from build123d import *

# Parameters (mm, degrees)
F1_DEPTH = 20
F3_DEPTH = 19.25
F5_DEPTH = 18
F6_W     = 10
F6_H     = 6
F6_H_2   = 4.5720012859
F7_DEPTH = 28.7263803184
F8_R     = 0.25
F9_R     = 0.5


with BuildPart() as f1:
    # F0 (on Top) → F1 (new body)
    with BuildSketch(Plane.XY):
        with BuildLine():
            ThreePointArc((47.25, 18.7263803184), (44.3210678119, 25.7974481303), (37.25, 28.7263803184))
            Line((37.25, 28.7263803184), (-37.25, 28.7263803184))
            ThreePointArc((-37.25, 28.7263803184), (-44.3210678119, 25.7974481303), (-47.25, 18.7263803184))
            Line((-47.25, 18.7263803184), (-47.25, -18.7263803184))
            ThreePointArc((-47.25, -18.7263803184), (-44.3210678119, -25.7974481303), (-37.25, -28.7263803184))
            Line((-37.25, -28.7263803184), (37.25, -28.7263803184))
            ThreePointArc((37.25, -28.7263803184), (44.3210678119, -25.7974481303), (47.25, -18.7263803184))
            Line((47.25, -18.7263803184), (47.25, 18.7263803184))
        make_face()
    extrude(amount=-F1_DEPTH)

    # F2 (on Top) → F3 (cut)
    with BuildSketch(Plane.XY):
        with BuildLine():
            Line((-45.25, 18.7263803184), (-45.25, -18.7263803184))
            ThreePointArc((-45.25, -18.7263803184), (-42.9068542495, -24.3832345679), (-37.25, -26.7263803184))
            Line((-37.25, -26.7263803184), (37.25, -26.7263803184))
            ThreePointArc((37.25, -26.7263803184), (42.9068542495, -24.3832345679), (45.25, -18.7263803184))
            Line((45.25, -18.7263803184), (45.25, 18.7263803184))
            ThreePointArc((45.25, 18.7263803184), (42.9068542495, 24.3832345679), (37.25, 26.7263803184))
            Line((37.25, 26.7263803184), (-37.25, 26.7263803184))
            ThreePointArc((-37.25, 26.7263803184), (-42.9068542495, 24.3832345679), (-45.25, 18.7263803184))
        make_face()
    extrude(amount=-F3_DEPTH, mode=Mode.SUBTRACT)

    # F4 (on face) → F5 (cut)
    with BuildSketch(Plane.XY.offset(-19.25)):
        with BuildLine():
            ThreePointArc((46.5, 18.7263803184), (43.790737726, 25.2671180444), (37.25, 27.9763803184))
            Line((37.25, 27.9763803184), (-37.25, 27.9763803184))
            ThreePointArc((-37.25, 27.9763803184), (-43.790737726, 25.2671180444), (-46.5, 18.7263803184))
            Line((-46.5, 18.7263803184), (-46.5, -18.7263803184))
            ThreePointArc((-46.5, -18.7263803184), (-43.790737726, -25.2671180444), (-37.25, -27.9763803184))
            Line((-37.25, -27.9763803184), (37.25, -27.9763803184))
            ThreePointArc((37.25, -27.9763803184), (43.790737726, -25.2671180444), (46.5, -18.7263803184))
            Line((46.5, -18.7263803184), (46.5, 18.7263803184))
        make_face()
    extrude(amount=F5_DEPTH, mode=Mode.SUBTRACT)

    # F6 (on Front) → F7 (cut, through all)
    with BuildSketch(Plane.XZ):
        with Locations((-21, -5)):
            Rectangle(F6_W, F6_H)
        with Locations((21, -4.2860006429)):
            Rectangle(F6_W, F6_H_2)
    extrude(amount=-F7_DEPTH, mode=Mode.SUBTRACT)

    # F8
    f8_edges = [f1.edges().sort_by_distance(p)[0] for p in [
        (-45.25, 0, 0),
        (-47.25, 0, 0),
        (-44.321068, 25.797448, 0),
        (-42.906854, 24.383235, 0),
        (0, 28.72638, 0),
        (0, 26.72638, 0),
        (44.321068, 25.797448, 0),
        (42.906854, 24.383235, 0),
        (47.25, 0, 0),
        (45.25, 0, 0),
        (44.321068, -25.797448, 0),
        (42.906854, -24.383235, 0),
        (0, -28.72638, 0),
        (0, -26.72638, 0),
        (-44.321068, -25.797448, 0),
        (-42.906854, -24.383235, 0),
        (-45.25, 0, -1.25),
        (-42.906854, 24.383235, -1.25),
        (0, 26.72638, -1.25),
        (42.906854, 24.383235, -1.25),
        (45.25, 0, -1.25),
        (0, -26.72638, -1.25),
        (42.906854, -24.383235, -1.25),
        (-42.906854, -24.383235, -1.25),
    ]]
    fillet(f8_edges, radius=F8_R)

    # F9
    f9_edges = [f1.edges().sort_by_distance(p)[0] for p in [
        (-44.321068, -25.797448, -20),
        (0, -28.72638, -20),
        (-47.25, 0, -20),
        (-44.321068, 25.797448, -20),
        (0, 28.72638, -20),
        (44.321068, 25.797448, -20),
        (47.25, 0, -20),
        (44.321068, -25.797448, -20),
        (-46.5, 0, -19.25),
        (-43.790738, 25.267118, -19.25),
        (0, 27.97638, -19.25),
        (43.790738, 25.267118, -19.25),
        (46.5, 0, -19.25),
        (43.790738, -25.267118, -19.25),
        (0, -27.97638, -19.25),
        (-43.790738, -25.267118, -19.25),
    ]]
    fillet(f9_edges, radius=F9_R)


solid = f1.part
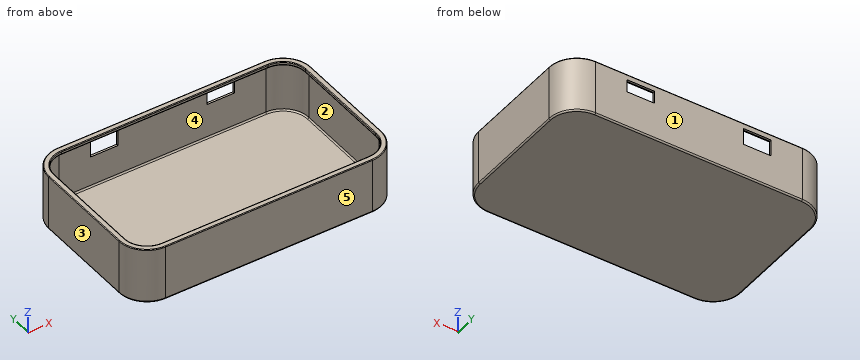
Design review of the part built by this model. Coordinates are the model's own, in mm. Face numbers are marked on the shaded views. A direction names the side the tool comes from. Coordinates: 2 decimals unless noted, no trailing zeros. Order: outer loops, then holes, each group sorted by start corner. A loop starts at its lowest first (then second) coordinate and runs counter-clockwise, first axis right, second up. Notation, with made-up numbers: M -27.75,57.5 L -17.75,57.5 A18 cw -17.75,87.5 Z; hole C -26,-10.75 d9. An arc over 180 degrees is marked long. Use a Markdown table: item, result.
(1) Add section D-D (x = -4). Give the boundary of the cut face in (y, z), then the cut area to 3 significant figures.
Worked answers:
| item | result |
|---|---|
| outline | M -28.73,-19.5 A0.5 ccw -28.23,-20 L 28.23,-20 A0.5 ccw 28.73,-19.5 L 28.73,-0.25 A0.25 ccw 28.48,0 L 26.98,0 A0.25 ccw 26.73,-0.25 L 26.73,-1 A0.25 ccw 26.98,-1.25 L 27.98,-1.25 L 27.98,-18.75 A0.5 cw 27.48,-19.25 L -27.48,-19.25 A0.5 cw -27.98,-18.75 L -27.98,-1.25 L -26.98,-1.25 A0.25 ccw -26.73,-1 L -26.73,-0.25 A0.25 ccw -26.98,0 L -28.48,0 A0.25 ccw -28.73,-0.25 Z |
| area | 75.0 mm2 |
(2) Add section C-C (y = 2). Give the boundary of the cut face in (x, z), then the cut area to 3 significant figures.
Worked answers:
| item | result |
|---|---|
| outline | M -47.25,-19.5 A0.5 ccw -46.75,-20 L 46.75,-20 A0.5 ccw 47.25,-19.5 L 47.25,-0.25 A0.25 ccw 47,0 L 45.5,0 A0.25 ccw 45.25,-0.25 L 45.25,-1 A0.25 ccw 45.5,-1.25 L 46.5,-1.25 L 46.5,-18.75 A0.5 cw 46,-19.25 L -46,-19.25 A0.5 cw -46.5,-18.75 L -46.5,-1.25 L -45.5,-1.25 A0.25 ccw -45.25,-1 L -45.25,-0.25 A0.25 ccw -45.5,0 L -47,0 A0.25 ccw -47.25,-0.25 Z |
| area | 103 mm2 |
(3) For the marked faces 4 and 5, list the 3-axis set-ups (+Z, -Z, +X, -X, +Y, -Y) from which the entire face can be reached by the end or side of a thin tool; tool diameter is ignored.
Worked answers:
| item | result |
|---|---|
| face 4 | none |
| face 5 | +Z, -Z, +X, -X, -Y |
(4) Add section A-A (x = 25). Give the boundary of the cut face in (y, z).
Worked answers:
| item | result |
|---|---|
| outline | M -28.73,-19.5 A0.5 ccw -28.23,-20 L 28.23,-20 A0.5 ccw 28.73,-19.5 L 28.73,-6.57 L 27.98,-6.57 L 27.98,-18.75 A0.5 cw 27.48,-19.25 L -27.48,-19.25 A0.5 cw -27.98,-18.75 L -27.98,-1.25 L -26.98,-1.25 A0.25 ccw -26.73,-1 L -26.73,-0.25 A0.25 ccw -26.98,0 L -28.48,0 A0.25 ccw -28.73,-0.25 Z; M 26.73,-1 A0.25 ccw 26.98,-1.25 L 27.98,-1.25 L 27.98,-2 L 28.73,-2 L 28.73,-0.25 A0.25 ccw 28.48,0 L 26.98,0 A0.25 ccw 26.73,-0.25 Z |
(5) Wall thickness on probe 1 along Y at (x, z) = (-13, -10.5); probe 2 along X at (y, z) = (-1, -5.25); probe 3 along Z at (x, y) = (-3.5, 16.5): over which ranges is each line inside the solid? List them lowest first.
Worked answers:
| item | result |
|---|---|
| probe 1 | y = -28.73 to -27.98, 27.98 to 28.73 |
| probe 2 | x = -47.25 to -46.5, 46.5 to 47.25 |
| probe 3 | z = -20 to -19.25 |
(6) Add section B-B (z = -12.25). Give the boundary of the cut face in (x, y).
Worked answers:
| item | result |
|---|---|
| outline | M -47.25,-18.73 A10 ccw -37.25,-28.73 L 37.25,-28.73 A10 ccw 47.25,-18.73 L 47.25,18.73 A10 ccw 37.25,28.73 L -37.25,28.73 A10 ccw -47.25,18.73 Z; hole M -46.5,-18.73 A9.25 ccw -37.25,-27.98 L 37.25,-27.98 A9.25 ccw 46.5,-18.73 L 46.5,18.73 A9.25 ccw 37.25,27.98 L -37.25,27.98 A9.25 ccw -46.5,18.73 Z |
(7) Draft analysis for pull direction X (two halves, no side actions). For the marked faces 1, 2 and 3, state which applies: released by +X, released by -X, zero draft, split by the parting line, or undercut.
Worked answers:
| item | result |
|---|---|
| face 1 | zero draft |
| face 2 | undercut |
| face 3 | released by -X |
(8) For P1, Ø0.8, axis at x = 19.5, y = 28.5, coming from the -Z side; P2, Ø16.5, axis at x = -20, y = 1, coming from the +Z side, all flat-tipped, find the tip position at first contact; note any pin that passes through.
Worked answers:
| item | result |
|---|---|
| P1 | stops at z = -20 |
| P2 | stops at z = -19.25 |
